Verification items for the finished model (mm, model axes). Face numbers are marked on the shaded views. A direction names the side the tool comes from. Give positions to 0.01 mm unless a question says otherwise; leave off trailing zeros. Order: outer loops, then holes, each group sorted by start corner. A loop starts at its lowest first (then second) coordinate and runs counter-clockwise, first axis right, second up. Notation, with made-up numbers: (18, -15.75) -> (34, -15.75) arc R35 ccw to (34, 18.25) -> close; hole circle Ø3 at (63, -32.5). An arc over 180 degrees is marked (long way). Return JSON: item names as keys, results as strings. Group by question number.
(1) Depth check by flat-ended pin: pin 1 Ø0.5 at (x, z) = (-1, 5) entering from +Y. Enter the tip coordinate at first touch or a pass-through.
(2) Cross-section at A-A on y = 2.6. Enter the section's corners in (x, z).
(3) Release check for a two-part mould opening along Y. For the marked faces 1 and 2 record: pulls with the +Y half, pulls with the -Y half, needs draft (parallel to the pull), parting line crosses it, or undercut.
(4) Tool access check on the marked faces 3 and 4. Record the directions out of +Z, -Z, +X, -X, +Y, -Y that give a thin tool (end or side, any length) a straight path to the whole face; none if there is none.
(5) Cross-section at C-C on x = 0.75. Enter the section's corners in (y, z), then the cut area to 3 significant figures.
(6) Thickness scan on line 1 along X through (y, z) = (4.9, 7); line 2 along Y through (x, z) = (-0.5, 7). Record the ranges inside material, lowest first.
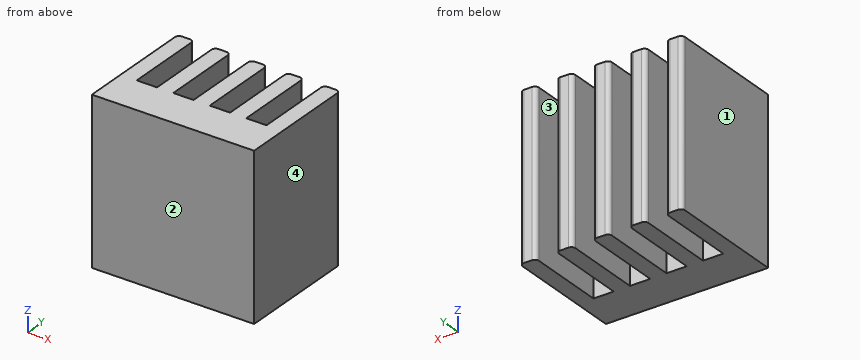
from build123d import *

# Parameters (mm, degrees)
BOSS_EXTRUDE1_DEPTH = 8
FILLET1_R           = 0.2


with BuildPart() as part:
    # Sketch1 → Boss-Extrude1 (new body)
    with BuildSketch(Plane.XY):
        Polygon((-4, 0), (4, 0), (4, 6), (3.2, 6), (3.2, 2), (2.2, 2), (2.2, 6), (1.4, 6), (1.4, 2), (0.4, 2), (0.4, 6), (-0.4, 6), (-0.4, 2), (-1.4, 2), (-1.4, 6), (-2.2, 6), (-2.2, 2), (-3.2, 2), (-3.2, 6), (-4, 6), align=None)
    extrude(amount=BOSS_EXTRUDE1_DEPTH)

    # Fillet1
    fillet1_edges = [part.edges().sort_by_distance(p)[0] for p in [
        (-4, 6, 4),
        (-3.2, 6, 4),
        (-2.2, 6, 4),
        (-1.4, 6, 4),
        (-0.4, 6, 4),
        (0.4, 6, 4),
        (1.4, 6, 4),
        (2.2, 6, 4),
        (3.2, 6, 4),
        (4, 6, 4),
    ]]
    fillet(fillet1_edges, radius=FILLET1_R)


solid = part.part
Verdict:
{
 "1": {"pin 1": "y = 2"},
 "2": {"outline": "(-4, 0) -> (-3.2, 0) -> (-3.2, 8) -> (-4, 8) -> close; (-2.2, 0) -> (-1.4, 0) -> (-1.4, 8) -> (-2.2, 8) -> close; (-0.4, 0) -> (0.4, 0) -> (0.4, 8) -> (-0.4, 8) -> close; (1.4, 0) -> (2.2, 0) -> (2.2, 8) -> (1.4, 8) -> close; (3.2, 0) -> (4, 0) -> (4, 8) -> (3.2, 8) -> close"},
 "3": {"face 1": "needs draft", "face 2": "pulls with the -Y half"},
 "4": {"face 3": "+Z, -Z, +Y", "face 4": "+Z, -Z, +X, +Y, -Y"},
 "5": {"outline": "(0, 0) -> (2, 0) -> (2, 8) -> (0, 8) -> close", "area": "16.0 mm²"},
 "6": {"line 1": "-4 to -3.2, -2.2 to -1.4, -0.4 to 0.4, 1.4 to 2.2, 3.2 to 4", "line 2": "0 to 2"}
}
